Read the model definition and answer for the solid it produces. Units are mm, in the model's axes. Coordinates: 2 decimals unless noted, no trailing zeros. Write each loop counter-clockwise with the first axis right and the second up, starting at its lowest first coordinate (ties: lowest second). Pieces come first, ordered by that corner, then holes.
(1) Given pin 1 (0.7 mm diameter, centred on x = 43, z = 14, fed in from -Y); pin 2 (0.7 mm diameter, centred on x = 39, z = 14, fed in from +Y), each flat-ended and moving along its own axis, determine where each tip first touches the part or whether it passes through.
(2) Section A-A on z = 14.15 is taken. Write down the section's boundary in (x, y), then the cut area to 3 significant figures.
(3) Section C-C on y = 6 is taken. Write down the section's boundary in (x, z), then the cut area to 3 significant figures.
(4) Find the intervals of material crossed by probe 1 along Y at (x, z) = (46, 13.45); probe 2 along X at (y, z) = (14, 13.9); probe 3 along X at (y, z) = (9.5, 13.45), in increasing order.
(5) Section B-B on x = 41.5 is taken. Write down the section's boundary in (y, z).
(6) Section D-D on y = -23.5 is taken. Write down the section's boundary in (x, z), then the cut area to 3 significant figures.
from build123d import *

# Parameters (mm, degrees)
BOSS_EXTRU_2_DEPTH = 1.3


with BuildPart() as part:
    # Esquisse2 → Boss.-Extru.2 (new body)
    with BuildSketch(Plane(origin=(0, 0, 14.509966587), x_dir=(-1, 0, 0), z_dir=(0, 0, -1))):
        Polygon((-55.223785445, -31.352276986), (-25.374778792, -43.716279214), (4.474220231, -31.352276986), (16.838222459, -1.503277963), (4.474220231, 28.345721061), (-25.374778792, 40.709719474), (-55.223785445, 28.345721061), (-67.587783858, -1.503277963), align=None)
        Polygon((-31.851776167, 10.053721244), (-31.851776167, -17.378277963), (-53.695785567, -17.378277963), (-53.695785567, 14.117724234), (-31.851776167, 14.117724234), (-31.851776167, 12.085718924), (-28.295776412, 12.085718924), (-28.295776412, 10.053721244), align=None, mode=Mode.SUBTRACT)
        with BuildLine():
            Line((-38.101776167, -21.860276406), (-39.529126769, -21.860276406))
            ThreePointArc((-39.529126769, -21.860276406), (-50.80118854, -24.813312469), (-39.4045428, -22.385089985))
            Line((-39.4045428, -22.385089985), (-38.101776167, -22.385089985))
            Line((-38.101776167, -22.385089985), (-38.101776167, -21.860276406))
        make_face(mode=Mode.SUBTRACT)
    extrude(amount=BOSS_EXTRU_2_DEPTH)


solid = part.part
Response:
1. pin 1: stops at y = -36.56
1. pin 2: stops at y = 35.21
2. outline: (-16.84, -1.5) - (-4.47, -31.35) - (25.37, -43.72) - (55.22, -31.35) - (67.59, -1.5) - (55.22, 28.35) - (25.37, 40.71) - (-4.47, 28.35) - close; hole (28.3, 10.05) - (31.85, 10.05) - (31.85, -17.38) - (53.7, -17.38) - (53.7, 14.12) - (31.85, 14.12) - (31.85, 12.09) - (28.3, 12.09) - close; hole (38.1, -22.39) - (39.4, -22.39) arc R5.83 ccw (long way) to (39.53, -21.86) - (38.1, -21.86) - close
2. area: 4,240 mm2
3. outline: (-13.73, 13.21) - (31.85, 13.21) - (31.85, 14.51) - (-13.73, 14.51) - close; (53.7, 13.21) - (64.48, 13.21) - (64.48, 14.51) - (53.7, 14.51) - close
3. area: 73.3 mm2
4. probe 1: y = -35.17 to -29.23, -17.7 to -17.38, 14.12 to 32.17
4. probe 2: x = -10.42 to 31.85, 53.7 to 61.17
4. probe 3: x = -12.28 to 31.85, 53.7 to 63.03
5. outline: (-37.04, 13.21) - (-28.03, 13.21) - (-28.03, 14.51) - (-37.04, 14.51) - close; (-18.91, 13.21) - (-17.38, 13.21) - (-17.38, 14.51) - (-18.91, 14.51) - close; (14.12, 13.21) - (34.03, 13.21) - (34.03, 14.51) - (14.12, 14.51) - close
6. outline: (-7.73, 13.21) - (39.3, 13.21) - (39.3, 14.51) - (-7.73, 14.51) - close; (50.96, 13.21) - (58.48, 13.21) - (58.48, 14.51) - (50.96, 14.51) - close
6. area: 70.9 mm2
